CAD build for the part. Positions are in the model's coordinates, mm. Give positions to 0.01 mm unless a question says otherwise; leave off trailing zeros. Order: outer loops, then holes, each group sorted by start corner. A loop starts at its lowest first (then second) coordinate and runs counter-clockwise, first axis right, second up.
Item 1: Band-saw the part on A-A on z = 12.7. Give the cut face in (x, y) (3 decimals).
Item 2: Two-plate mould, pull along X, no slides. Class faces 1 (the cylindrical face through (-66.53, 6.44, 13.65)), 2 (the flat face through (2, 6, 0)), 3 (the flat face through (-127, 6, 13)): released by +X, released by -X, zero draft, split by the parting line, or undercut.
Item 3: Band-saw the part on B-B on x = -63.5. Give the cut face in (y, z) (3 decimals), plus the area to 3 significant figures.
Item 4: Wall check: L1, parallel to X at y = 10.75, z = 13; L2, parallel to Z at x = 63.5, y = 5 (3 decimals); L3, parallel to X at y = 6.5, z = 13.75. Give the ranges that are in metal, low to high.
Item 5: Flat gauge pin, fed straight in: P1, Ø4, axis at x = 63.5, z = 12.7, coming from the +Y side. Where does the tip first touch, or does it go through?
```python
from build123d import *

# Parameters (mm, degrees)
F0_W          = 12.7
F0_H          = 25.4
F1_DEPTH      = 127
F1_DEPTH_BACK = 127
F3_D          = 6.35


with BuildPart() as f1:
    # F0 (on Right) → F1 (new body, two sides)
    with BuildSketch(Plane.YZ) as f1_sk:
        with Locations((6.35, 12.7)):
            Rectangle(F0_W, F0_H)
    extrude(amount=F1_DEPTH)
    extrude(f1_sk.sketch, amount=-F1_DEPTH_BACK)

    # F3 (through all)
    with Locations(Plane.XZ):
        with Locations((-63.5, 12.7), (63.5, 12.7)):
            Hole(F3_D / 2)


solid = f1.part
```
The answers:
1. outline: (-127, 0) - (-66.675, 0) - (-66.675, 12.7) - (-127, 12.7) - close; (-60.325, 0) - (60.325, 0) - (60.325, 12.7) - (-60.325, 12.7) - close; (66.675, 0) - (127, 0) - (127, 12.7) - (66.675, 12.7) - close
2. face 1: undercut
2. face 2: zero draft
2. face 3: released by -X
3. outline: (0, 0) - (12.7, 0) - (12.7, 9.525) - (0, 9.525) - close; (0, 15.875) - (12.7, 15.875) - (12.7, 25.4) - (0, 25.4) - close
3. area: 242 mm2
4. L1: x = -127 to -66.66, -60.34 to 60.34, 66.66 to 127
4. L2: z = 0 to 9.525, 15.875 to 25.4
4. L3: x = -127 to -66.5, -60.5 to 60.5, 66.5 to 127
5. P1: passes through
